```python
from build123d import *

# Parameters (mm, degrees)
SKETCH2_W           = 22
SKETCH2_H           = 12.5
SKETCH2_R           = 2.425
BOSS_EXTRUDE1_DEPTH = 15
SKETCH3_R           = 1.755
CUT_EXTRUDE1_DEPTH  = 30
FILLET1_R           = 2.5


with BuildPart() as part:
    # Sketch2 → Boss-Extrude1 (new body)
    with BuildSketch(Plane.XY):
        with Locations((0, 18.75)):
            Rectangle(SKETCH2_W, SKETCH2_H)
        with Locations((-6.25, 20.5)):
            Circle(SKETCH2_R, mode=Mode.SUBTRACT)
        with Locations((6.25, 20.5)):
            Circle(SKETCH2_R, mode=Mode.SUBTRACT)
    extrude(amount=BOSS_EXTRUDE1_DEPTH)

    # Sketch3 → Cut-Extrude1 (cut)
    with BuildSketch(Plane(origin=(11, 0, 0), x_dir=(0, 0, -1), z_dir=(1, 0, 0))):
        with Locations((-10, 15)):
            Circle(SKETCH3_R)
    extrude(amount=-CUT_EXTRUDE1_DEPTH, mode=Mode.SUBTRACT)

    # Fillet1
    fillet1_edges = [part.edges().sort_by_distance(p)[0] for p in [
        (-11, 25, 7.5),
        (11, 25, 7.5),
    ]]
    fillet(fillet1_edges, radius=FILLET1_R)


solid = part.part
```
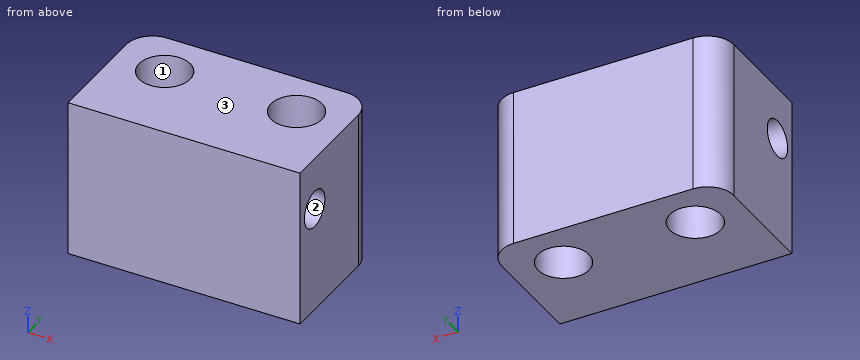
Here's how the part is built. I have some questions about the finished solid (model axes, mm). Face numbers are marked on the shaded views. Give positions to 0.01 mm unless a question says otherwise; leave off trailing zeros. Loops run counter-clockwise (first coordinate to the right, second up) from the corner with the lowest first, then second, coordinate; pieces in that order, holes last. Notation, with made-up numbers: M 84,9.25 L 125,9.25 A21 ccw 125,38.25 Z; hole C 87,37 d9. An arc over 180 degrees is marked long. Put each result on its own line as item: value. Start each with the question number.
(1) Will these pins go through, and if not, where does the flat tip stop? pin 1 Ø1 at (y, z) = (23.5, 2.5) entering from -X; pin 2 Ø5.5 at (x, y) = (-6.25, 20.5) entering from -Z; pin 3 Ø3 at (y, z) = (15, 10) entering from -X.
(2) I want a section at D-D on y = 20.5. Please give me the cut outline in (x, z) (3 decimals), then the cut area to 4 significant figures.
(3) I want a section at A-A on z = 10. Please give me the cut outline in (x, y) (3 decimals).
(4) I want a section at C-C on y = 15. Please give me the cut outline in (x, z) (3 decimals), then the cut area to 3 significant figures.
(5) I need wall thicknesses on line 1 along Y through (x, z) = (-6.25, 10) (3 decimals); line 2 along Y through (x, z) = (6.25, 5.5) (3 decimals); line 3 along Y through (x, z) = (2.5, 10) (3 decimals). Which ranges of each line are inside material? Lowest first, please. Write a range as [from, to].
(6) I want a section at B-B on x = -6.25. Please give me the cut outline in (y, z) (3 decimals), then the cut area to 3 significant figures.
(7) If we mould it in two halves opening along Z, with no side actions, what happens to the marked faces 1, 2 and 3? For each: +Z half, -Z half, draft (parallel to the pull), parting line (faces both ways), or undercut.
Answer block:
1. pin 1: x = -10.95
1. pin 2: z = 0
1. pin 3: through
2. outline: M -11,0 L -8.675,0 L -8.675,15 L -11,15 Z; M -3.825,0 L 3.825,0 L 3.825,15 L -3.825,15 Z; M 8.675,0 L 11,0 L 11,15 L 8.675,15 Z
2. area: 184.5 mm^2
3. outline: M -11,12.5 L 11,12.5 L 11,13.245 L -11,13.245 Z; M -11,16.755 L 11,16.755 L 11,22.5 A2.5 ccw 8.5,25 L -8.5,25 A2.5 ccw -11,22.5 Z; hole C -6.25,20.5 d4.85; hole C 6.25,20.5 d4.85
4. outline: M -11,0 L 11,0 L 11,8.245 L -11,8.245 Z; M -11,11.755 L 11,11.755 L 11,15 L -11,15 Z
4. area: 253 mm^2
5. line 1: [12.5, 13.245], [16.755, 18.075], [22.925, 25]
5. line 2: [12.5, 18.075], [22.925, 25]
5. line 3: [12.5, 13.245], [16.755, 25]
6. outline: M 12.5,0 L 18.075,0 L 18.075,15 L 12.5,15 Z; M 22.925,0 L 25,0 L 25,15 L 22.925,15 Z; hole C 15,10 d3.51
6. area: 105 mm^2
7. face 1: draft
7. face 2: undercut
7. face 3: +Z half
